```python
from build123d import *

# Parameters (mm, degrees)
MODEL_W             = 17.8592
MODEL_H             = 44.1523
BOSS_EXTRUDE1_DEPTH = 3
SKETCH2_R           = 0.8509
CUT_EXTRUDE1_DEPTH  = 48.721867314


with BuildPart() as part:
    # Model → Boss-Extrude1 (new body)
    with BuildSketch(Plane.XY):
        with Locations((8.9296, 22.07615)):
            Rectangle(MODEL_W, MODEL_H)
        Polygon((8.9296, 24.03615), (9.324632213, 23.934630441), (9.72680382, 23.866699097), (10.046391979, 23.613282289), (10.386163858, 23.387645988), (10.575048267, 23.02615), (10.793670772, 22.681823309), (10.819191601, 22.27475408), (10.878862915, 21.871274212), (10.736607381, 21.489017711), (10.627009791, 21.09615), (10.341575168, 20.804801848), (10.081659094, 20.490476691), (9.702399622, 20.34041363), (9.337106914, 20.158980703), (8.9296, 20.17615), (8.522093086, 20.158980703), (8.156800378, 20.34041363), (7.777540906, 20.490476691), (7.517624832, 20.804801848), (7.232190209, 21.09615), (7.122592619, 21.489017711), (6.980337085, 21.871274212), (7.040008399, 22.27475408), (7.065529228, 22.681823309), (7.284151733, 23.02615), (7.473036142, 23.387645988), (7.812808021, 23.613282289), (8.13239618, 23.866699097), (8.534567787, 23.934630441), align=None, mode=Mode.SUBTRACT)
    extrude(amount=BOSS_EXTRUDE1_DEPTH)

    # Sketch2 → Cut-Extrude1 (cut, through all)
    with BuildSketch(Plane.XY.offset(3)):
        with Locations((8.9296, 6.83615)):
            Circle(SKETCH2_R)
        with Locations(Location((8.9296, 37.31615, 0), (0, 0, 180))):
            Circle(SKETCH2_R)
    extrude(amount=-CUT_EXTRUDE1_DEPTH, mode=Mode.SUBTRACT)


solid = part.part
```
Build history of the part. All positions in model axes, mm. Round coordinates to 2 decimals unless told otherwise and drop trailing zeros. Put each result on its own line as item: value.
Item 1: Wall check: probe 1 along Y at (x, z) = (9, 0.75); probe 2 along Y at (x, z) = (8.5, 0.5); probe 3 along X at (y, z) = (20.5, 0.5). Give the ranges that are in metal, low to high. Write a range as from..to.
Here are the results:
probe 1: y = 0..5.99, 7.68..20.17, 24.02..36.47, 38.16..44.15
probe 2: y = 0..6.1, 7.57..20.17, 23.93..36.58, 38.05..44.15
probe 3: x = 0..7.77, 10.09..17.86
Item 2: Two-plate mould, pull along X, no slides. Class faces 1 (the face through (17.859, 22, 1)), 2 (the face through (9.716, 6.51, 1.521)), 3 (the face through (8.144, 37.642, 1.521)), 4 (the face through (9, 44.152, 1)): pulls with the +X half, pulls with the -X half, needs draft (parallel to the pull), parting line crosses it, or undercut.
Here are the results:
face 1: pulls with the +X half
face 2: undercut
face 3: undercut
face 4: needs draft
Item 3: Flat gauge pins, fed straight in: P1, Ø1, axis at x = 8.93, y = 37.32, coming from the -Z side; P2, Ø10, axis at x = 2, y = 17.5, coming from the -Z side. Where does each tip first touch, or does it go through?
Here are the results:
P1: passes through
P2: stops at z = 0
Item 4: Slice it at A-A, the plane z = 1.6. Count the separate pieces of the cut face and the enclosed holes in it, plus the area to 3 significant figures.
Here are the results:
separate pieces: 1
enclosed holes: 3
area: 772 mm^2
